For this review, take the finished solid that the model builds, in its own axes (mm). A direction names the side the tool comes from. Round coordinates to 2 decimals unless told otherwise and drop trailing zeros. Order: outer loops, then holes, each group sorted by start corner. A loop starts at its lowest first (then second) coordinate and runs counter-clockwise, first axis right, second up. Notation, with made-up numbers: (81, -8) - (118, -8) arc R29 cw to (118, 23) - close; hole circle Ø9 at (25, -21). An arc over 180 degrees is marked (long way). One line per question, with ' | ' between items.
```python
from build123d import *

# Parameters (mm, degrees)
SKETCH1_W           = 22
SKETCH1_H           = 17.5
BOSS_EXTRUDE1_DEPTH = 1.925
SKETCH2_R           = 0.4064
FILLET1_R           = 0.5


with BuildPart() as part:
    # Sketch1 → Boss-Extrude1 (new, symmetric)
    with BuildSketch(Plane(origin=(0, 0, 0), x_dir=(0, 0, -1), z_dir=(1, 0, 0))):
        Rectangle(SKETCH1_W, SKETCH1_H)
    extrude(amount=BOSS_EXTRUDE1_DEPTH, both=True)

    # Sweep1: sweep along a path in Sketch3
    with BuildLine(Plane.XY.offset(10)) as sweep1_path:
        Line((0, -8.75), (0, -9.588170614))
        Line((0, -9.588170614), (-0.118311478, -9.793092105))
    # Sketch2 → Sweep1 (sweep)
    with BuildSketch(Plane.XZ.offset(8.75)):
        with Locations((0, 10)):
            Circle(SKETCH2_R)
    sweep1 = sweep(path=sweep1_path.line, transition=Transition.RIGHT)

    # Fillet1
    fillet1_edges = [part.edges().sort_by_distance(p)[0] for p in [
        (1.925, 0, 11),
        (1.925, -8.75, 0),
        (1.925, 0, -11),
        (-1.925, -8.75, 0),
        (-1.925, 0, 11),
        (-1.925, 8.75, 0),
        (-1.925, 0, -11),
        (0, -8.75, -11),
        (0, -8.75, 11),
        (0, 8.75, 11),
        (0, 8.75, -11),
        (1.925, 8.75, 0),
    ]]
    fillet(fillet1_edges, radius=FILLET1_R)

    # Mirror1: Sweep1 across plane
    add(sweep1.mirror(Plane.XY))


solid = part.part
```
(1) Mouldability with a two-part tool opening along Z and no side actions: class faces 1 (the flat face through (0, 0, 11)), 2 (the flat face through (0, -8.75, 0)), 3 (the flat face through (-1.925, 0, 0)) as released by +Z, released by -Z, zero draft, split by the parting line, or undercut.
Output values:
face 1: released by +Z | face 2: undercut | face 3: zero draft
(2) For probe 1 along Y at (x, z) = (1.4, -9.5); probe 2 along Z at (x, y) = (1.5, 3.5); probe 3 along Z at (x, y) = (1.75, 3), list the stretches that pass through material, from the lowest coordinate up. Write a range as [from, to].
Output values:
probe 1: [-8.75, 8.75] | probe 2: [-10.99, 10.99] | probe 3: [-10.88, 10.88]
(3) We need section B-B on x = -0.95. State the section outline as (y, z) points.
Output values:
outline: (-8.75, -10.5) arc R0.5 ccw to (-8.25, -11) - (8.25, -11) arc R0.5 ccw to (8.75, -10.5) - (8.75, 10.5) arc R0.5 ccw to (8.25, 11) - (-8.25, 11) arc R0.5 ccw to (-8.75, 10.5) - close
(4) We need section C-C on z = 10. State the section outline as (x, y) points (3 decimals), plus the area to 3 significant figures.
Output values:
outline: (-1.925, -8.25) arc R0.5 ccw to (-1.425, -8.75) - (-0.406, -8.75) - (-0.406, -9.479) - (-0.47, -9.59) - (0.234, -9.996) - (0.406, -9.697) - (0.406, -8.75) - (1.425, -8.75) arc R0.5 ccw to (1.925, -8.25) - (1.925, 8.25) arc R0.5 ccw to (1.425, 8.75) - (-1.425, 8.75) arc R0.5 ccw to (-1.925, 8.25) - close | area: 68.0 mm^2
(5) For faces 4 (the flat face through (0, 0, -11)), 5 (the cylindrical face through (0.375, -9.125, -9.844)), list the 3-axis set-ups (+Z, -Z, +X, -X, +Y, -Y) from which the entire face can be reached by the end or side of a thin tool; tool diameter is ignored.
Output values:
face 4: -Z, +X, -X, +Y, -Y | face 5: none
(6) We need section A-A on z = 3. State the section outline as (x, y) points (3 decimals).
Output values:
outline: (-1.925, -8.25) arc R0.5 ccw to (-1.425, -8.75) - (1.425, -8.75) arc R0.5 ccw to (1.925, -8.25) - (1.925, 8.25) arc R0.5 ccw to (1.425, 8.75) - (-1.425, 8.75) arc R0.5 ccw to (-1.925, 8.25) - close
